Autodesk Inventor part; units mm, degrees
ref_plane "YZ Plane" through (0, 0, 0) normal (1, 0, 0) x (0, 1, 0)
ref_plane "XZ Plane" through (0, 0, 0) normal (0, 1, 0) x (-1, 0, 0)
ref_plane "XY Plane" through (0, 0, 0) normal (0, 0, 1) x (1, 0, 0)
sketch "スケッチ1" plane through (0, 0, 0) normal (0, 1, 0) x (-1, 0, 0)
  circle A0 centre (-0.0357, -0.0516) radius 12.5
  circle A1 centre (-0.0357, -0.0516) radius 5
  circle A2 centre (-0.0357, -0.0516) radius 3.5
  circle A3 centre (-0.0357, -0.0516) radius 9
  arc A4 (-9.0357, -0.0516) -> (4.4643, -7.8458) centre (-0.0357, -0.0516) ccw
  line L0 (-0.0357, -0.0516) -> (4.4643, -7.8458) construction
  line L1 (-0.0357, -0.0516) -> (-9.0357, -0.0516) construction
  arc A5 (4.4643, 7.7426) -> (-9.0357, -0.0516) centre (-0.0357, -0.0516) ccw
  line L2 (-0.0357, -0.0516) -> (4.4643, 7.7426) construction
  line L3 (-0.0357, -0.0516) -> (-9.0357, -0.0516) construction
  line L4 (-9.0357, -0.0516) -> (-9.0357, 0.9484)
  line L5 (-9.0357, -0.0516) -> (-8.0357, -0.0516) construction
  line L6 (-9.0357, 0.9484) -> (-4.9347, 0.9484)
  line L7 (-9.0357, -0.0516) -> (-9.0357, -1.0516)
  line L8 (-9.0357, -0.0516) -> (-8.0357, -0.0516) construction
  line L9 (-9.0357, -1.0516) -> (-4.9347, -1.0516)
  line L10 (4.4643, 7.7426) -> (3.5983, 8.2426)
  line L11 (4.4643, 7.7426) -> (5.4643, 7.7426) construction
  line L12 (1.5477, 4.691) -> (3.5983, 8.2426)
  line L13 (4.4643, 7.7426) -> (5.3012, 7.1953)
  line L14 (5.3012, 7.1953) -> (3.2798, 3.691)
  line L15 (4.4643, -7.8458) -> (3.5983, -8.3458)
  line L16 (4.4643, -7.8458) -> (5.4643, -7.8458) construction
  line L17 (3.5983, -8.3458) -> (1.5477, -4.7942)
  line L18 (4.4643, -7.8458) -> (5.3303, -7.3458)
  line L19 (4.4643, -7.8458) -> (5.4643, -7.8458) construction
  line L20 (5.3303, -7.3458) -> (3.2798, -3.7942)
  circle A6 centre (-0.0357, -0.0516) radius 12
  point P0 (0, 0)
  point P1 (-9.0357, -0.0516)
  point P2 (3.5704, -8.2976)
  point P3 (-8.98, -1.0516)
  point P4 (-8.98, 0.9484)
  point P5 (3.5704, 8.1944)
  point P6 (5.3024, -7.2976)
  dimension "d1" = 25
  dimension "d2" = 10
  dimension "d3" = 7
  dimension "d4" = 18
  dimension "d5" = 120
  dimension "d6" = 120
  dimension "d7" = 1
  dimension "d8" = 90
  dimension "d9" = 1
  dimension "d10" = 90
  dimension "d11" = 1
  dimension "d12" = 150
  dimension "d13" = 1
  dimension "d14" = 1
  dimension "d15" = 150
  dimension "d16" = 1
  dimension "d17" = 30
  dimension "d18" = 24
extrude "押し出し1" add sketch "スケッチ1" along normal blind 12 contours A0
extrude "押し出し2" add sketch "スケッチ1" along normal blind 1 contours A1 L12 A3 L13 L14 | L20 A3 L17 A1 | L13 A3 | L20 L18 A3 | A1 L9 A3 L6 | L12 L10 A3 | A3 L15 L17 | A3 L4 L6 | L9 L7 A3 | A6
extrude "押し出し3" add sketch "スケッチ1" along normal blind 3 contours A1
extrude "押し出し4" add sketch "スケッチ1" against normal blind 1 from surface at 12 contours A1 | A1 L12 A3 L13 L14 | L20 A3 L17 A1 | L13 A3 | L20 L18 A3 | A1 L9 A3 L6 | L12 L10 A3 | A3 L15 L17 | A3 L4 L6 | L9 L7 A3 | A6
extrude "押し出し5" add sketch "スケッチ1" along normal blind 2 from surface at 12 contours A1
sketch "スケッチ2" plane through (0.0357, 12, -0.0516) normal (0, 1, 0) x (1, 0, 0)
  circle A0 centre (0, 0) radius 9.5
  arc A1 (-4.75, -8.2272) -> (9.5, 0) centre (0, 0) ccw
  line L0 (0, 0) -> (-4.75, -8.2272) construction
  line L1 (0, 0) -> (9.5, 0) construction
  arc A2 (9.5, 0) -> (-4.75, 8.2272) centre (0, 0) ccw
  line L2 (0, 0) -> (-4.75, 8.2272) construction
  line L3 (0, 0) -> (9.5, 0) construction
  circle A3 centre (9.5, 0) radius 1
  circle A4 centre (-4.75, -8.2272) radius 1
  circle A5 centre (-4.75, 8.2272) radius 1
  point P0 (-0.0357, -0.0516)
  dimension "d29" = 19
  dimension "d30" = 120
  dimension "d31" = 120
  dimension "d32" = 2
  dimension "d33" = 2
  dimension "d34" = 2
extrude "押し出し6" add sketch "スケッチ2" along normal blind 2 contours A0 A3 | A0 A3 | A5 A0 | A0 A5 | A4 A0 | A0 A4
equation "\"BendRadius\" = Thickness"
equation "\"BendReliefWidth\" = Thickness"
equation "\"BendReliefDepth\" = 0.5 * Thickness"
equation "\"CornerReliefSize\" = 4 * Thickness"
equation "\"MinimumRemnant\" = 2 * Thickness"
equation "\"TransitionRadius\" = BendRadius"
equation "\"JacobiRadiusSize\" = BendRadius"
equation "\"GapSize\" = Thickness"
properties part number "RobTrace_Wheel" material "ABS プラスチック"
Model file for the job. Use its own axes, mm. A direction names the side the tool comes from. Give positions to 0.01 mm unless a question says otherwise; leave off trailing zeros. Order: outer loops, then holes, each group sorted by start corner. A loop starts at its lowest first (then second) coordinate and runs counter-clockwise, first axis right, second up.
1) Pin check, flat tips, straight feed: pin 1 (2 mm diameter, centred on x = 4.5, y = 7, fed in from -Z); pin 2 (1.5 mm diameter, centred on x = -5, y = 8.5, fed in from +Z); pin 3 (5 mm diameter, centred on x = -3.5, y = 11.5, fed in from +Z). Stop position of each tip, or through.
2) Saw through at B-B, the plane z = -3. Count the separate pieces of the cut face and the enclosed holes in it, then the cut area to 3 significant figures.
3) Wall check: probe 1 along Y at (x, z) = (10.5, 4.5); probe 2 along Y at (x, z) = (-3.75, 0.25); probe 3 along Z at (x, y) = (4.25, 7.5). Give the ranges that are in metal, low to high.
4) Saw through at A-A, the plane y = 13. Write the cut outline in (x, z).
5) Saw through at D-D, the plane z = 6.25. Write the cut outline in (x, y), then the cut area to 3 significant figures.
6) Mould opens along Z. For faces 1 (the cylindrical face through (-11.887, 5.916, -3.806)), 2 (the flat face through (-4.305, 0.493, -5.57)), 3 (the cylindrical face through (4.433, 0.493, -7.904)), 4 (the flat face through (10, 14, 0)) say: +Z half, -Z half, draft (parallel to the pull), parting line (faces both ways), or undercut.
7) 3-axis set-ups, long thin cutter, end or side, ignore diameter. For faces 5 (the flat face through (-2.1, 3, -3.3)), 6 (the flat face through (-2.545, 0.493, 6.418)), 7 (the flat face through (6, 12, 0)): which of +Z, -Z, +X, -X, +Y, -Y reach the whole face in a straight line?
8) Saw through at C-C, the plane x = 11. Write the cut outline in (y, z), then the cut area to 3 significant figures.
Computed:
1. pin 1: stops at z = -12.06
1. pin 2: stops at z = 11.69
1. pin 3: stops at z = 12.41
2. separate pieces: 6
2. enclosed holes: 0
2. area: 50.7 mm2
3. probe 1: y = 0 to 1, 11 to 12
3. probe 2: y = 0 to 3, 11 to 14
3. probe 3: z = -11.82 to -11.29, 11.18 to 11.72
4. outline: circle Ø2 at (-4.71, -8.28); circle Ø2 at (-4.71, 8.18); circle Ø10 at (0.04, -0.05); circle Ø2 at (9.54, -0.05); hole circle Ø7 at (0.04, -0.05)
5. outline: (-10.76, 0) - (-6.39, 0) - (-6.39, 1) - (-10.18, 1) - (-10.18, 11) - (-6.39, 11) - (-6.39, 12) - (-10.76, 12) - close; (-4.76, 0) - (-2.45, 0) - (-2.45, 1) - (-4.76, 1) - close; (-4.76, 11) - (-2.45, 11) - (-2.45, 12) - (-4.76, 12) - close; (6.46, 0) - (10.83, 0) - (10.83, 12) - (6.46, 12) - (6.46, 11) - (10.25, 11) - (10.25, 1) - (6.46, 1) - close
5. area: 33.8 mm2
6. face 1: parting line
6. face 2: undercut
6. face 3: undercut
6. face 4: draft
7. face 5: none
7. face 6: +Y, -Y
7. face 7: +Y
8. outline: (0, -6.05) - (12, -6.05) - (12, 5.95) - (0, 5.95) - close; hole (1, -4.93) - (11, -4.93) - (11, 4.83) - (1, 4.83) - close
8. area: 46.5 mm2
